Geometry: final body of the model. Coordinates: model frame, mm. A direction names the side the tool comes from. Give positions to 0.01 mm unless a question says otherwise; leave off trailing zeros. Loops run counter-clockwise (first coordinate to the right, second up) from the corner with the lowest first, then second, coordinate; pieces in that order, holes last.
1. Material intervals for line 1 along Y through (x, z) = (-16, 12); line 2 along X through (y, z) = (-12.5, 8.75); line 3 along X through (y, z) = (-12, 5), sorted ascending.
2. Draft query along X for faces 1 (the face through (6.265, -41.412, -13.075)), 2 (the face through (22.5, -42, 0)), 3 (the face through (-16.08, -72.86, 1.06)), 4 (the face through (14, -41, -16.5)). Return one class per face: +X half, -X half, draft (parallel to the pull), parting line (faces both ways), or undercut.
3. Section B-B, the plane x = 0. Output: boundary loops of the cut face in (y, z).
4. Section A-A, the plane y = -43. Output: boundary loops of the cut face in (x, z) (3 decimals), then the cut area to 3 significant figures.
5. Access query for faces 5 (the face through (17.666, -73.778, 9.199)), 6 (the face through (-6.53, -84.7, -12.97)), 7 (the face through (-15, -41, -16.5)). Directions: +Z, -Z, +X, -X, +Y, -Y. A direction counts if a zero-diameter tool reaches every point of the face in a straight line with its end or side. Return the directions, or none.
6. First-contact query: P1, Ø9.5, axis at x = 0, z = -3.5, coming from the -Y side; P2, Ø2.5, axis at x = -16, y = -72.5, coming from the +Z side; P3, Ø3.5, axis at x = -16, y = -12.5, coming from the +Z side; P4, Ø1.5, axis at x = 3, y = -47.5, coming from the -Z side. Flat tips, straight axial feed; report the tip coordinate or a pass-through.
from build123d import *

# Parameters (mm, degrees)
F1_DEPTH = 85
F2_R     = 1
F4_D     = 4.2
F4_DEPTH = 14.4
F4_TIP   = 1.2618073


with BuildPart() as f1:
    # F0 (on Front) → F1 (new body)
    with BuildSketch(Plane.XZ):
        with BuildLine():
            Line((22.5, 16.5), (-22.5, 16.5))
            Line((-22.5, 16.5), (-22.5, -16.5))
            Line((-22.5, -16.5), (-7.5654657558, -16.5))
            Line((-7.5654657558, -16.5), (-5, -9.7449979984))
            ThreePointArc((-5, -9.7449979984), (0, 4.5), (5, -9.7449979984))
            Line((5, -9.7449979984), (7.5654657558, -16.5))
            Line((7.5654657558, -16.5), (22.5, -16.5))
            Line((22.5, -16.5), (22.5, 16.5))
        make_face()
    extrude(amount=F1_DEPTH)

    # F2
    f2_edges = [f1.edges().sort_by_distance(p)[0] for p in [
        (-22.5, -42.5, 16.5),
        (-22.5, -42.5, -16.5),
        (-22.5, 0, 0),
        (-22.5, -85, 0),
        (22.5, -42.5, 16.5),
        (0, 0, 16.5),
        (0, -85, 16.5),
        (-15.032733, -85, -16.5),
        (-6.282733, -85, -13.122499),
        (0, -85, 4.5),
        (6.282733, -85, -13.122499),
        (15.032733, -85, -16.5),
        (22.5, -85, 0),
        (22.5, -42.5, -16.5),
        (22.5, 0, 0),
    ]]
    fillet(f2_edges, radius=F2_R)

    # F4
    with Locations(Plane.XY.offset(16.5)):
        with Locations((-16, -12.5), (16, -12.5), (-16, -72.5), (16, -72.5)):
            Hole(F4_D / 2, depth=F4_DEPTH)
            with Locations((0, 0, -(F4_DEPTH + F4_TIP / 2))):  # 118° drill point
                Cone(0, F4_D / 2, F4_TIP, mode=Mode.SUBTRACT)


solid = f1.part
Answers below:
1. line 1: y = -85 to -74.6, -70.4 to -14.6, -10.4 to 0
1. line 2: x = -22.5 to -18.1, -13.9 to 13.9, 18.1 to 22.5
1. line 3: x = -22.5 to -18.04, -13.96 to 13.96, 18.04 to 22.5
2. face 1: undercut
2. face 2: +X half
2. face 3: undercut
2. face 4: draft
3. outline: (-85, 5.5) arc R1 ccw to (-84, 4.5) - (0, 4.5) - (0, 15.5) arc R1 ccw to (-1, 16.5) - (-84, 16.5) arc R1 ccw to (-85, 15.5) - close
4. outline: (-22.5, -15.5) arc R1 ccw to (-21.5, -16.5) - (-7.565, -16.5) - (-5, -9.745) arc R8 cw (long way) to (5, -9.745) - (7.565, -16.5) - (21.5, -16.5) arc R1 ccw to (22.5, -15.5) - (22.5, 15.5) arc R1 ccw to (21.5, 16.5) - (-21.5, 16.5) arc R1 ccw to (-22.5, 15.5) - close
4. area: 1,210 mm2
5. face 5: +Z
5. face 6: -Z, -Y
5. face 7: -Z, +X, -X, +Y, -Y
6. P1: passes through
6. P2: stops at z = 1.59
6. P3: stops at z = 1.89
6. P4: stops at z = 3.57
